Geometry check sheet. Reference: the model listing, model coordinates, mm. Face numbers are marked on the shaded views. A direction names the side the tool comes from. Round coordinates to 2 decimals unless told otherwise and drop trailing zeros. Loops run counter-clockwise (first coordinate to the right, second up) from the corner with the lowest first, then second, coordinate; pieces in that order, holes last.
```python
from build123d import *

# Parameters (mm, degrees)
BOX003_W     = 3
BOX003_H     = 1.5
BOX003_DEPTH = 2
BOX001_W     = 6
BOX001_H     = 3.5
BOX001_DEPTH = 4.5
BOX002_W     = 7
BOX002_H     = 4.5
BOX002_DEPTH = 8


with BuildPart() as cube002:
    # Box003 → Box003 (new body)
    with BuildSketch(Plane(origin=(12.5, 13, 10), x_dir=(1, 0, 0), z_dir=(0, 0, 1))):
        with Locations((1.5, 0.75)):
            Rectangle(BOX003_W, BOX003_H)
    extrude(amount=BOX003_DEPTH)


with BuildPart() as cube:
    # Box001 → Box001 (new body)
    with BuildSketch(Plane(origin=(11, 12, 1.6), x_dir=(1, 0, 0), z_dir=(0, 0, 1))):
        with Locations((3, 1.75)):
            Rectangle(BOX001_W, BOX001_H)
    extrude(amount=BOX001_DEPTH)


with BuildPart() as obj1:
    # Box002 → Box002 (new body)
    with BuildSketch(Plane(origin=(10.5, 11.5, 2), x_dir=(1, 0, 0), z_dir=(0, 0, 1))):
        with Locations((3.5, 2.25)):
            Rectangle(BOX002_W, BOX002_H)
    extrude(amount=BOX002_DEPTH)

    # Cut: cut Cube
    add(cube.part, mode=Mode.SUBTRACT)

    # Fusion: union Cube002
    add(cube002.part)


solid = obj1.part
```
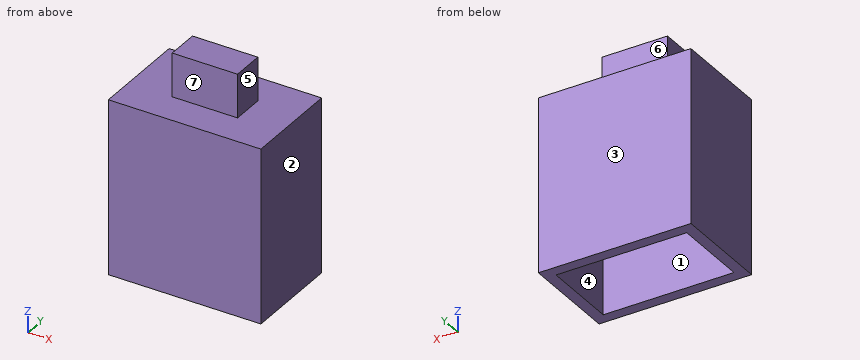
1) Mould release check, pull along X, two halves, no side actions. Record for the marked faces 1, 2, 3 and 4: +X half, -X half, draft (parallel to the pull), parting line (faces both ways), or undercut.
Report:
face 1: undercut
face 2: +X half
face 3: draft
face 4: undercut
2) Sectioned sample at C-C, the plane y = 12.3. Record the cut outline in (x, z).
Report:
outline: (10.5, 2) - (11, 2) - (11, 6.1) - (17, 6.1) - (17, 2) - (17.5, 2) - (17.5, 10) - (10.5, 10) - close
3) Gauge pin test, flat ends, axial feed: pin 1 (2 mm diameter, centred on x = 13.5, z = 11.5, fed in from +Y); pin 2 (0.6 mm diameter, centred on x = 14.5, z = 11, fed in from -Y); pin 3 (1.2 mm diameter, centred on y = 13.5, z = 11, fed in from -X). Record the tip position at first contact, or that the pin passes through.
Report:
pin 1: stops at y = 14.5
pin 2: stops at y = 13
pin 3: stops at x = 12.5
4) Scan lines: line 1 along X through (y, z) = (14.5, 2.5); line 2 along Y through (x, z) = (12.25, 6); line 3 along Z through (x, y) = (14.5, 12.1). Record each from-to range of solid material in increasing order.
Report:
line 1: x = 10.5 to 11, 17 to 17.5
line 2: y = 11.5 to 12, 15.5 to 16
line 3: z = 6.1 to 10
5) Access from +Z, -Z, +X, -X, +Y, -Y to the whole of each face (thin tool, end or side, straight path). Record for the marked faces 5, 6 and 7.
Report:
face 5: +Z, +X, +Y, -Y
face 6: +Z, +X, -X, +Y
face 7: +Z, +X, -X, -Y
6) Sectioned sample at D-D, the plane z = 11.25. Record the cut outline in (x, y), then the cut area to 3 significant figures.
Report:
outline: (12.5, 13) - (15.5, 13) - (15.5, 14.5) - (12.5, 14.5) - close
area: 4.50 mm2
7) Sectioned sample at A-A, the plane z = 3.5. Record the cut outline in (x, y), then the cut area to 3 significant figures.
Report:
outline: (10.5, 11.5) - (17.5, 11.5) - (17.5, 16) - (10.5, 16) - close; hole (11, 12) - (17, 12) - (17, 15.5) - (11, 15.5) - close
area: 10.5 mm2
8) Sectioned sample at B-B, the plane x = 16.5. Record the cut outline in (y, z).
Report:
outline: (11.5, 2) - (12, 2) - (12, 6.1) - (15.5, 6.1) - (15.5, 2) - (16, 2) - (16, 10) - (11.5, 10) - close
